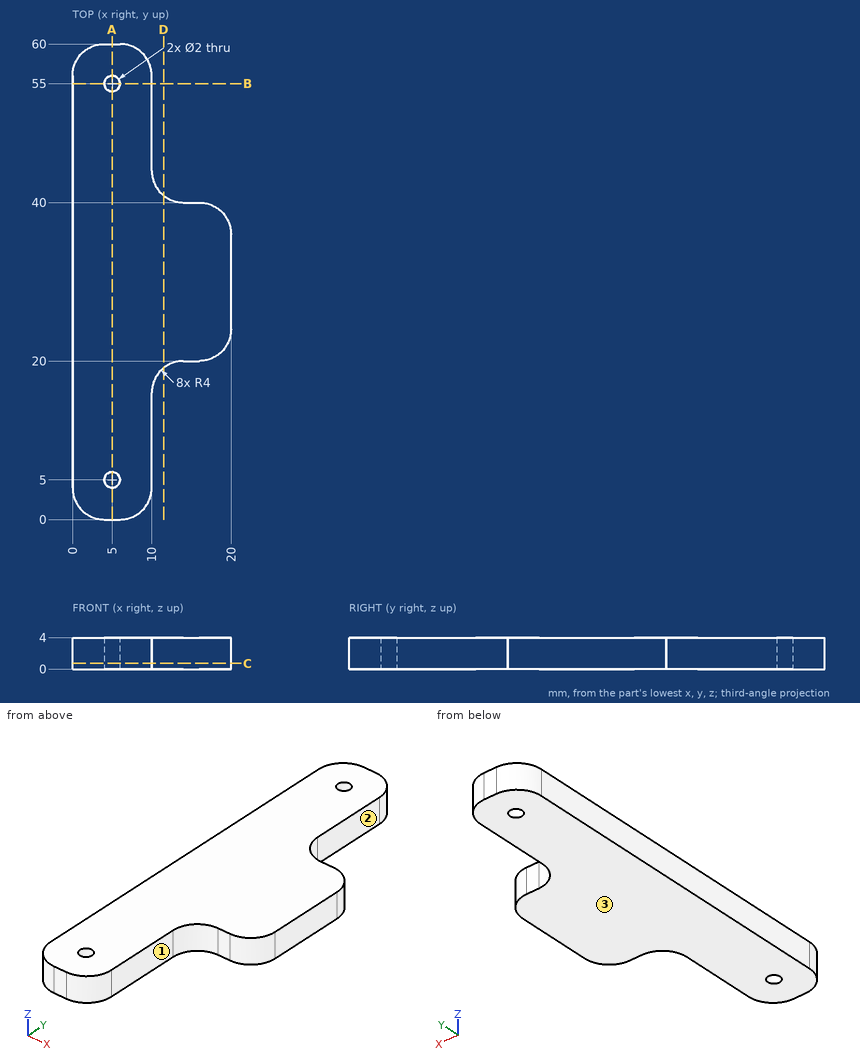
Can you work these out from the drawing? Everything is in mm from the part's minimum corner. A direction names the side the tool comes from. Round coordinates to 2 decimals unless told otherwise and drop trailing zeros. Write each loop counter-clockwise with the first axis right and the second up, starting at its lowest first coordinate (ties: lowest second). Pieces come first, ordered by that corner, then holes. Notation, with made-up numbers: (-14.75, 43) - (18.25, 43) arc R14 ccw to (18.25, 59) - close; hole circle Ø4 at (43.25, 65.5). An arc over 180 degrees is marked (long way). Put each result on its own line as item: value. Start each with the question number.
(1) I want a section at A-A, the plane x = 5. Please give me the cut outline in (y, z), plus the area to 3 significant figures.
(2) For the marked faces 1, 2 and 3, which set-ups out of +Z, -Z, +X, -X, +Y, -Y let a thin tool reach every point of the face, with its end or its side?
(3) I want a section at B-B, the plane y = 55. Please give me the cut outline in (x, z).
(4) I need wall thicknesses on probe 1 along Y at (x, z) = (5, 2); probe 2 along X at (y, z) = (55, 2.85); probe 3 along X at (y, z) = (12.5, 0.75). Which ranges of each line are inside material? Lowest first, please.
(5) Will these pins go through, and if not, where does the flat tip stop? pin 1 (0.6 mm diameter, centred on x = 15.5, z = 1.5, fed in from -Y); pin 2 (1 mm diameter, centred on x = 15.5, z = 2, fed in from +Y).
(6) I want a section at C-C, the plane z = 0.75. Please give me the cut outline in (x, y).
(7) I want a section at D-D, the plane x = 11.5. Please give me the cut outline in (y, z).
Here are the results:
1. outline: (0, 0) - (4, 0) - (4, 4) - (0, 4) - close; (6, 0) - (54, 0) - (54, 4) - (6, 4) - close; (56, 0) - (60, 0) - (60, 4) - (56, 4) - close
1. area: 224 mm^2
2. face 1: +Z, -Z, +X, -Y
2. face 2: +Z, -Z, +X, +Y
2. face 3: -Z, +X, -X, +Y, -Y
3. outline: (0, 0) - (4, 0) - (4, 4) - (0, 4) - close; (6, 0) - (10, 0) - (10, 4) - (6, 4) - close
4. probe 1: y = 0 to 4, 6 to 54, 56 to 60
4. probe 2: x = 0 to 4, 6 to 10
4. probe 3: x = 0 to 10
5. pin 1: stops at y = 20
5. pin 2: stops at y = 40
6. outline: (0, 4) arc R4 ccw to (4, 0) - (6, 0) arc R4 ccw to (10, 4) - (10, 16) arc R4 cw to (14, 20) - (16, 20) arc R4 ccw to (20, 24) - (20, 36) arc R4 ccw to (16, 40) - (14, 40) arc R4 cw to (10, 44) - (10, 56) arc R4 ccw to (6, 60) - (4, 60) arc R4 ccw to (0, 56) - close; hole circle Ø2 at (5, 5); hole circle Ø2 at (5, 55)
7. outline: (19.12, 0) - (40.88, 0) - (40.88, 4) - (19.12, 4) - close
